```python
from build123d import *

# Parameters (mm, degrees)
SKETCH1_W               = 66.04
SKETCH1_H               = 101.6
BASE_EXTRUDE_DEPTH      = 2.54
SKETCH2_W               = 73.66
SKETCH2_H               = 109.22
SKETCH2_W_2             = 66.04
SKETCH2_H_2             = 101.6
WALLS_DEPTH             = 25.4
BUTTON_GUIDE_DEPTH      = 22.86
SKETCH4_R               = 1.3
CUT_EXTRUDE1_DEPTH      = 129.502413207
HARD_STOP_DEPTH         = 7.62
SKETCH6_W               = 9.144
SKETCH6_H               = 3.81
SKETCH6_W_2             = 10.668
SKETCH6_H_2             = 7.62
ELECTRONICS_HOLES_DEPTH = 19.05
FILLET1_R               = 2.54
SKETCH7_W               = 10.16
SKETCH7_H               = 5.08
BOSS_EXTRUDE1_DEPTH     = 10.16
SKETCH8_W               = 10.16
SKETCH8_H               = 5.08
BOSS_EXTRUDE2_DEPTH     = 10.16
SKETCH9_R               = 3.302
CUT_EXTRUDE2_DEPTH      = 138.406722543
FILLET2_R               = 2.54


with BuildPart() as part:
    # Sketch1 → Base Extrude (new body)
    with BuildSketch(Plane(origin=(0, 0, 0), x_dir=(1, 0, 0), z_dir=(0, 1, 0))):
        with Locations((33.02, 50.8)):
            Rectangle(SKETCH1_W, SKETCH1_H)
    extrude(amount=BASE_EXTRUDE_DEPTH)

    # Sketch2 → Walls (add)
    with BuildSketch(Plane.XZ):
        with Locations((33.02, -50.8)):
            Rectangle(SKETCH2_W, SKETCH2_H)
        with Locations((33.02, -50.8)):
            Rectangle(SKETCH2_W_2, SKETCH2_H_2, mode=Mode.SUBTRACT)
    extrude(amount=-WALLS_DEPTH)

    # Sketch3 → Button Guide (add)
    with BuildSketch(Plane(origin=(0, 25.4, 0), x_dir=(1, 0, 0), z_dir=(0, 1, 0))):
        Polygon((3.81, 86.36), (0, 84.583367822), (0, 76.2), (3.81, 76.2), align=None)
        Polygon((18.543367822, 101.6), (0, 101.6), (0, 93.216632178), (3.81, 91.44), (3.81, 97.79), (20.32, 97.79), align=None)
        Polygon((66.04, 101.6), (27.176632178, 101.6), (25.4, 97.79), (62.23, 97.79), (62.23, 91.44), (66.04, 93.216632178), align=None)
        Polygon((66.04, 76.2), (66.04, 84.583367822), (62.23, 86.36), (62.23, 76.2), align=None)
    extrude(amount=-BUTTON_GUIDE_DEPTH)

    # Sketch4 → Cut-Extrude1 (cut, through all)
    with BuildSketch(Plane(origin=(0, 2.54, 0), x_dir=(1, 0, 0), z_dir=(0, 1, 0))):
        with Locations(Location((8.0645, 92.542598833, 0), (0, 0, 270))):
            Circle(SKETCH4_R)
        with Locations(Location((57.9755, 92.542598833, 0), (0, 0, 270))):
            Circle(SKETCH4_R)
        with Locations(Location((8.0645, 7.452598833, 0), (0, 0, 270))):
            Circle(SKETCH4_R)
        with Locations(Location((57.9755, 7.452598833, 0), (0, 0, 270))):
            Circle(SKETCH4_R)
    extrude(amount=-CUT_EXTRUDE1_DEPTH, mode=Mode.SUBTRACT)

    # Sketch5 → Hard stop (add)
    with BuildSketch(Plane(origin=(0, 2.54, 0), x_dir=(1, 0, 0), z_dir=(0, 1, 0))):
        Polygon((0, 93.216632178), (0, 84.583367822), (3.81, 86.36), (3.81, 91.44), align=None)
        Polygon((18.543367822, 101.6), (27.176632178, 101.6), (25.4, 97.79), (20.32, 97.79), align=None)
        Polygon((62.23, 91.44), (66.04, 93.216632178), (66.04, 84.583367822), (62.23, 86.36), align=None)
    extrude(amount=HARD_STOP_DEPTH)

    # Sketch6 → Electronics Holes (cut)
    with BuildSketch(Plane(origin=(0, 25.4, 0), x_dir=(1, 0, 0), z_dir=(0, 1, 0))):
        with Locations((42.418, -1.905)):
            Rectangle(SKETCH6_W, SKETCH6_H)
        with Locations((42.3545, 101.6)):
            Rectangle(SKETCH6_W_2, SKETCH6_H_2)
    extrude(amount=-ELECTRONICS_HOLES_DEPTH, mode=Mode.SUBTRACT)

    # Fillet1
    fillet1_edges = [part.edges().sort_by_distance(p)[0] for p in [
        (37.846, 6.35, 1.905),
        (46.99, 6.35, 1.905),
    ]]
    fillet(fillet1_edges, radius=FILLET1_R)

    # Sketch7 → Boss-Extrude1 (add)
    with BuildSketch(Plane.XY.offset(3.81)):
        with Locations((13.97, 22.86)):
            Rectangle(SKETCH7_W, SKETCH7_H)
    extrude(amount=BOSS_EXTRUDE1_DEPTH)

    # Sketch8 → Boss-Extrude2 (add)
    with BuildSketch(Plane(origin=(0, 0, -105.41), x_dir=(-1, 0, 0), z_dir=(0, 0, -1))):
        with Locations((-13.97, 22.86)):
            Rectangle(SKETCH8_W, SKETCH8_H)
    extrude(amount=BOSS_EXTRUDE2_DEPTH)

    # Sketch9 → Cut-Extrude2 (cut, through all)
    with BuildSketch(Plane(origin=(0, 25.4, 0), x_dir=(1, 0, 0), z_dir=(0, 1, 0))):
        with Locations(Location((13.97, 110.49, 0), (0, 0, 270))):
            Circle(SKETCH9_R)
        with Locations(Location((13.97, -8.89, 0), (0, 0, 270))):
            Circle(SKETCH9_R)
    extrude(amount=-CUT_EXTRUDE2_DEPTH, mode=Mode.SUBTRACT)

    # Fillet2
    fillet2_edges = [part.edges().sort_by_distance(p)[0] for p in [
        (8.89, 22.86, 3.81),
        (19.05, 22.86, 3.81),
        (8.89, 22.86, 13.97),
        (19.05, 22.86, 13.97),
        (19.05, 22.86, -105.41),
        (8.89, 22.86, -105.41),
        (19.05, 22.86, -115.57),
        (8.89, 22.86, -115.57),
    ]]
    fillet(fillet2_edges, radius=FILLET2_R)


solid = part.part
```
The listing builds one solid part. Answer for the finished solid, in the listing's coordinates (mm). A direction names the side the tool comes from. Give positions to 0.01 mm unless a question says otherwise; leave off trailing zeros. Write each loop counter-clockwise with the first axis right and the second up, starting at its lowest first coordinate (ties: lowest second). Pieces come first, ordered by that corner, then holes. Notation, with made-up numbers: M 32,26 L 47,26 A10 ccw 47,42 Z; hole C -8.75,4 d10. An arc over 180 degrees is marked long. Write each question's results on one line, items separated by ' | '.
Q1. Consider L1, parallel to X at y = 12.75, z = -87.5; L2, parallel to X at y = 9.5, z = 1; L3, parallel to Z at x = 48.5, y = 12. Determine where each line is inside the solid, lowest interval first. Write a range as from..to.
Output values:
L1: -3.81..0, 66.04..69.85 | L2: -3.81..37.85, 46.99..69.85 | L3: -105.41..-97.79, 0..3.81
Q2. For a pull along X with two mould halves and no side action, classify faces 4 (the flat face through (42, 6.35, -102)), 5 (the flat face through (-3.81, 13, -52)), 6 (the flat face through (33, 0, -50)) as released by +X, released by -X, zero draft, split by the parting line, or undercut.
Output values:
face 4: undercut | face 5: released by -X | face 6: zero draft
Q3. Section A-A, the plane z = -110.49 is taken. Write down the section's boundary in (x, y).
Output values:
outline: M 8.89,20.32 L 10.67,20.32 L 10.67,25.4 L 8.89,25.4 Z; M 17.27,20.32 L 19.05,20.32 L 19.05,25.4 L 17.27,25.4 Z
Q4. Section C-C, the plane y = 23 is taken. Count the separate pieces of the cut face and the enclosed holes in it, then the cut area to 3 significant figures.
Output values:
separate pieces: 2 | enclosed holes: 2 | area: 1,700 mm2
Q5. A tool of negligible diameter and unlimited length cuts with its end or side. For faces 1 (the flat face through (0, 14, -39)), 2 (the flat face through (47.689, 16, -102)), 3 (the cylindrical face through (38.57, 7.114, 1.878)), from which of +Z, -Z, +X, -X, +Y, -Y can it reach the whole face along a straight path? Write none if from no direction.
Output values:
face 1: +Y | face 2: -Z, +Y | face 3: +Z, -Z, +Y
Q6. Flat-ended cylindrical pins translate along their axes: P1, Ø4, axis at x = 55.5, y = 13.5, coming from the -Z side; P2, Ø1.5, axis at x = 8.5, z = -34, coming from the +Y side; P3, Ø1.9, axis at x = 1, z = -91, coming from the +Y side; P4, Ø4, axis at x = 13.97, z = 8.89, coming from the +Y side. Find the tip coordinate at first contact, or state that the pin passes through.
Output values:
P1: z = -105.41 | P2: y = 2.54 | P3: y = 10.16 | P4: through
Q7. Section B-B, the plane x = 13.97 is taken. Write down the section's boundary in (y, z), then the cut area to 3 significant figures.
Output values:
outline: M 0,-105.41 L 20.32,-105.41 L 20.32,-107.19 L 25.4,-107.19 L 25.4,-97.79 L 2.54,-97.79 L 2.54,0 L 25.4,0 L 25.4,5.59 L 20.32,5.59 L 20.32,3.81 L 0,3.81 Z; M 20.32,-115.57 L 25.4,-115.57 L 25.4,-113.79 L 20.32,-113.79 Z; M 20.32,12.19 L 25.4,12.19 L 25.4,13.97 L 20.32,13.97 Z | area: 575 mm2
Q8. Section D-D, the plane z = -56 is taken. Write down the section's boundary in (x, y), then the cut area to 3 significant figures.
Output values:
outline: M -3.81,0 L 69.85,0 L 69.85,25.4 L 66.04,25.4 L 66.04,2.54 L 0,2.54 L 0,25.4 L -3.81,25.4 Z | area: 361 mm2
